Design review of the part built by this model. Coordinates are the model's own, in mm. Face numbers are marked on the shaded views. Coordinates: 2 decimals unless noted, no trailing zeros. Loops run counter-clockwise (first coordinate to the right, second up) from the corner with the lowest first, then second, coordinate; pieces in that order, holes last.
from build123d import *

# Parameters (mm, degrees)
SKETCH1_W             = 40
SKETCH1_H             = 88
SKETCH1_R             = 2.5
BOSS_EXTRUDE1_DEPTH   = 5
SKETCH2_R             = 7
SKETCH2_R_2           = 4.15
BOSS_EXTRUDE2_DEPTH   = 20
CHAMFER1_SIZE         = 10
CHAMFER1_SIZE2        = 0.174550649
CHAMFER1_PART_2_SIZE  = 10
CHAMFER1_PART_2_SIZE2 = 0.174550649
FILLET1_R             = 5


with BuildPart() as part:
    # Sketch1 → Boss-Extrude1 (new body)
    with BuildSketch(Plane(origin=(0, 0, 0), x_dir=(1, 0, 0), z_dir=(0, 1, 0))):
        Rectangle(SKETCH1_W, SKETCH1_H)
        with Locations((-14, 38)):
            Circle(SKETCH1_R, mode=Mode.SUBTRACT)
        with Locations((14, 38)):
            Circle(SKETCH1_R, mode=Mode.SUBTRACT)
        with Locations((-14, 12)):
            Circle(SKETCH1_R, mode=Mode.SUBTRACT)
        with Locations((14, 12)):
            Circle(SKETCH1_R, mode=Mode.SUBTRACT)
        with Locations((-14, -12)):
            Circle(SKETCH1_R, mode=Mode.SUBTRACT)
        with Locations((-14, -38)):
            Circle(SKETCH1_R, mode=Mode.SUBTRACT)
        with Locations((14, -38)):
            Circle(SKETCH1_R, mode=Mode.SUBTRACT)
        with Locations((14, -12)):
            Circle(SKETCH1_R, mode=Mode.SUBTRACT)
    extrude(amount=BOSS_EXTRUDE1_DEPTH)

    # Sketch2 → Boss-Extrude2 (add)
    with BuildSketch(Plane(origin=(0, 0, 0), x_dir=(1, 0, 0), z_dir=(0, 1, 0))):
        with Locations((0, 25)):
            Circle(SKETCH2_R)
        with Locations((0, 25)):
            Circle(SKETCH2_R_2, mode=Mode.SUBTRACT)
        with Locations((0, -25)):
            Circle(SKETCH2_R)
        with Locations((0, -25)):
            Circle(SKETCH2_R_2, mode=Mode.SUBTRACT)
    extrude(amount=BOSS_EXTRUDE2_DEPTH)

    # Chamfer1
    chamfer1_edges = [part.edges().sort_by_distance(p)[0] for p in [
        (-4.15, 5, 25),
    ]]
    chamfer1_side = [part.faces().sort_by_distance(p)[0] for p in [
        (-4.15, 12.5, 25),
    ]]
    chamfer(chamfer1_edges, length=CHAMFER1_SIZE, length2=CHAMFER1_SIZE2, reference=chamfer1_side[0])

    # Chamfer1 part 2
    chamfer1_part_2_edges = [part.edges().sort_by_distance(p)[0] for p in [
        (-4.15, 5, -25),
    ]]
    chamfer1_part_2_side = [part.faces().sort_by_distance(p)[0] for p in [
        (-4.15, 12.5, -25),
    ]]
    chamfer(chamfer1_part_2_edges, length=CHAMFER1_PART_2_SIZE, length2=CHAMFER1_PART_2_SIZE2, reference=chamfer1_part_2_side[0])

    # Fillet1
    fillet1_edges = [part.edges().sort_by_distance(p)[0] for p in [
        (-7, 5, 25),
        (-7, 5, -25),
        (-20, 2.5, -44),
        (20, 2.5, -44),
        (20, 2.5, 44),
        (-20, 2.5, 44),
    ]]
    fillet(fillet1_edges, radius=FILLET1_R)


solid = part.part
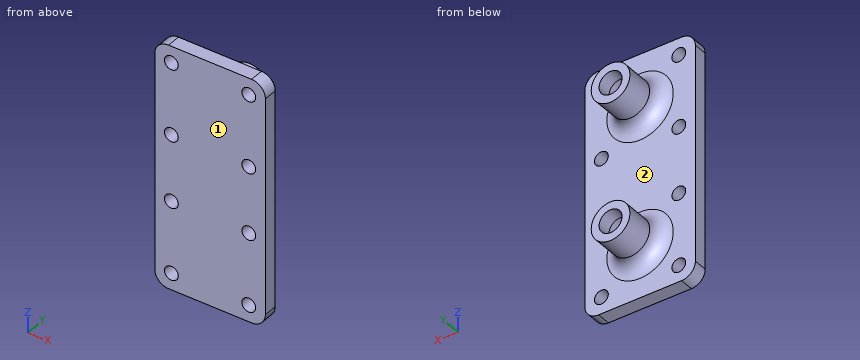
Q1. Take a section at B-B, the plane z = 12. Write out the cut boundary in (x, y), then the cut area to 3 significant figures.
Q2. Take a section at C-C, the plane y = 8.25. Write out the cut boundary in (x, z).
Q3. Clearance check with flat-ended pins moving along their axes: pin 1 Ø8 at (x, z) = (-1.5, -2.5) entering from +Y; pin 2 Ø6 at (y, z) = (12.5, 16.5) entering from -X; pin 3 Ø1.5 at (y, z) = (9, 21) entering from -X (3 decimals). State where each tip first meets the part, or that it passes through.
Q4. The part is to be moulded in two halves that separate along Z. For the marked faces 1 and 2, say which applies: pulls with the +Z half, pulls with the -Z half, needs draft (parallel to the pull), parting line crosses it, or undercut.
Q5. For line 1 (Z direction, x = -14, y = 4.25); line 2 (X direction, y = 1.6, z = 38); line 3 (Z direction, x = 0, y = 17.3), list the stretches that pass through material, from the lowest coordinate up.
Q6. Take a section at D-D, the plane z = 1. Write out the cut boundary in (x, y), then the cut area to 3 significant figures.
Q7. Take a section at A-A, the plane x = 14. Write out the cut boundary in (y, z), then the cut area to 3 significant figures.
Entries:
1. outline: (-20, 0) - (-16.5, 0) - (-16.5, 5) - (-20, 5) - close; (-11.5, 0) - (11.5, 0) - (11.5, 5) - (-11.5, 5) - close; (16.5, 0) - (20, 0) - (20, 5) - (16.5, 5) - close
1. area: 150 mm2
2. outline: circle Ø14.63 at (0, -25); circle Ø14.63 at (0, 25); hole circle Ø8.06 at (0, -25); hole circle Ø8.06 at (0, 25)
3. pin 1: stops at y = 5
3. pin 2: stops at x = -4.33
3. pin 3: stops at x = -6.365
4. face 1: needs draft
4. face 2: undercut
5. line 1: z = -44 to -40.5, -35.5 to -14.5, -9.5 to 9.5, 14.5 to 35.5, 40.5 to 44
5. line 2: x = -20 to -16.5, -11.5 to 11.5, 16.5 to 20
5. line 3: z = -32 to -29.15, -20.85 to -18, 18 to 20.85, 29.15 to 32
6. outline: (-20, 0) - (20, 0) - (20, 5) - (-20, 5) - close
6. area: 200 mm2
7. outline: (0, -44) - (5, -44) - (5, -40.5) - (0, -40.5) - close; (0, -35.5) - (5, -35.5) - (5, -14.5) - (0, -14.5) - close; (0, -9.5) - (5, -9.5) - (5, 9.5) - (0, 9.5) - close; (0, 14.5) - (5, 14.5) - (5, 35.5) - (0, 35.5) - close; (0, 40.5) - (5, 40.5) - (5, 44) - (0, 44) - close
7. area: 340 mm2
